Source: CAD feature listing. Evaluate the final solid. Frame: model axes, mm. Face numbers are marked on the shaded views. A direction names the side the tool comes from. Coordinates: 2 decimals unless noted, no trailing zeros. Order: outer loops, then holes, each group sorted by start corner. A loop starts at its lowest first (then second) coordinate and runs counter-clockwise, first axis right, second up.
Item 1: Contact query for flat-ended pins moving along their axis: P1, Ø6, axis at x = -8.5, z = 5.5, coming from the -Y side; P2, Ø3.5, axis at x = -0.5, y = -8, coming from the +Z side. Output: stop coordinate, or through.
Item 2: Section A-A on x = -0.75. Return the cut outline in (y, z), then the cut area to 3 significant figures.
Item 3: Ray query, line 1 (Z direction, x = 7, y = -9); line 2 (Y direction, x = -8, z = -39). Return the intervals inside material, ascending.
Item 4: Section C-C on z = 17. Return the cut outline in (x, y), then the cut area to 3 significant figures.
Item 5: Reachability of the marked faces 1 and 2 from +Z, -Z, +X, -X, +Y, -Y: full face, straight path, thin tool, end or side. Return the list, or none.
Item 6: Section B-B on y = -8.25. Return the cut outline in (x, z), then the cut area to 3 significant figures.
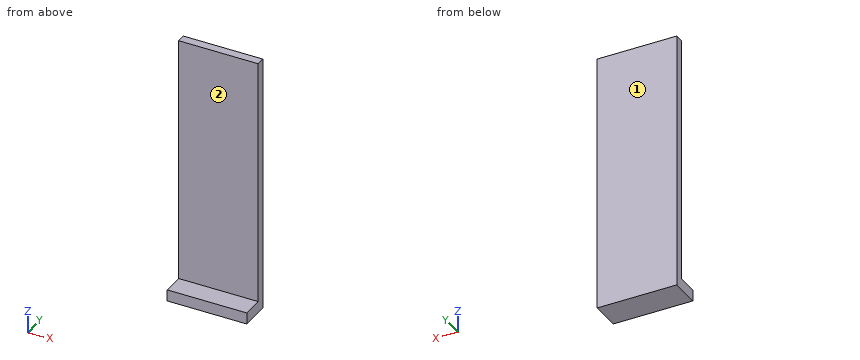
from build123d import *

# Parameters (mm, degrees)
F0_W     = 27.5
F0_H     = 90
F1_DEPTH = 3
F2_W     = 27.5
F2_H     = 10.3
F3_DEPTH = 4


with BuildPart() as f1:
    # F0 (on Front) → F1 (new body)
    with BuildSketch(Plane.XZ):
        with Locations((0, -5)):
            Rectangle(F0_W, F0_H)
    extrude(amount=F1_DEPTH)

    # F2 (on face) → F3 (join)
    with BuildSketch(Plane(origin=(0, 0, -50), x_dir=(1, 0, 0), z_dir=(0, 0, -1))):
        with Locations((0, 5.15)):
            Rectangle(F2_W, F2_H)
    extrude(amount=-F3_DEPTH)


solid = f1.part
Answer list:
1. P1: stops at y = -3
1. P2: stops at z = -46
2. outline: (-10.3, -50) - (0, -50) - (0, 40) - (-3, 40) - (-3, -46) - (-10.3, -46) - close
2. area: 299 mm2
3. line 1: z = -50 to -46
3. line 2: y = -3 to 0
4. outline: (-13.75, -3) - (13.75, -3) - (13.75, 0) - (-13.75, 0) - close
4. area: 82.5 mm2
5. face 1: +Z, -Z, +X, -X, +Y
5. face 2: +Z, +X, -X, -Y
6. outline: (-13.75, -50) - (13.75, -50) - (13.75, -46) - (-13.75, -46) - close
6. area: 110 mm2
